Input: part model. Units: mm. Frame: model coordinates. A direction names the side the tool comes from. Coordinates: 2 decimals unless noted, no trailing zeros. Use CSV: the item, a comma, the result in double quotes.
```python
from build123d import *

# Parameters (mm, degrees)
F0_W     = 25.4
F0_H     = 25.4
F1_DEPTH = 25.4
F2_R     = 12.69999


# Not quite as in the source:
# - a fillet or chamfer is up to 0.001 mm smaller than in the source, because OpenCascade refuses the exact size


with BuildPart() as f1:
    # F0 (on Front) → F1 (new body)
    with BuildSketch(Plane.XZ):
        Polygon((-30.9433350532, 41.3746904978), (-56.3433350532, 41.3746904978), (-56.3433350532, -9.4253095022), (-30.9433350532, -9.4253095022), (-30.9433350532, 15.9746904978), align=None)
        with Locations((-18.2433350532, 28.6746904978)):
            Rectangle(F0_W, F0_H)
    extrude(amount=F1_DEPTH)

    # F2 (radius 12.7 in the source; OpenCascade refuses exactly that, so slightly less here)
    f2_edges = [f1.edges().sort_by_distance(p)[0] for p in [
        (-56.343335, 0, 15.97469),
        (-56.343335, -25.4, 15.97469),
        (-30.943335, -25.4, 41.37469),
        (-56.343335, -12.7, 41.37469),
        (-30.943335, 0, 41.37469),
        (-18.243335, -25.4, 15.97469),
        (-30.943335, -25.4, 3.27469),
        (-30.943335, 0, 3.27469),
        (-18.243335, 0, 15.97469),
        (-30.943335, -12.7, 15.97469),
    ]]
    fillet(f2_edges, radius=F2_R)


solid = f1.part
```
1. Contact query for flat-ended pins moving along their axis: pin 1 Ø4 at (y, z) = (-14.5, 9) entering from -X; pin 2 Ø10 at (x, z) = (-24, 16.5) entering from +Y; pin 3 Ø5 at (x, z) = (-20, 14.5) entering from +Y; pin 4 Ø1.5 at (x, y) = (-23, -4.5) entering from +Z. Output: stop coordinate, or through.
Resolved:
pin 1,"stops at x = -56.34"
pin 2,"stops at y = -1.49"
pin 3,"stops at y = -7.39"
pin 4,"stops at z = 38.96"
2. Material intervals for line 1 (Z direction, x = -28.5, y = -3.75); line 2 (X direction, y = -19, z = 12.5); line 3 (Y direction, x = -50.5, z = 21.5), sorted ascending. Write a range as [from, to].
Resolved:
line 1,"z = [16.06, 37.69]"
line 2,"x = [-54.67, -29.26]"
line 3,"y = [-23.39, -2.01]"
3. Access query for faces 1 (the cylindrical face through (-24.86, -3.819, 37.753)), 2 (the cylindrical face through (-11.804, -3.819, 19.596)), 3 (the cylindrical face through (-34.565, -21.581, -2.986)). Directions: +Z, -Z, +X, -X, +Y, -Y. A direction counts if a zero-diameter tool reaches every point of the face in a straight line with its end or side. Return the directions, or none.
Resolved:
face 1,"+Z, +X, -X, +Y"
face 2,"-Z, +X, +Y"
face 3,"-Z, +X, -Y"
